Geometry check sheet. Reference: the model listing, model coordinates, mm. Give positions to 0.01 mm unless a question says otherwise; leave off trailing zeros. Write each loop counter-clockwise with the first axis right and the second up, starting at its lowest first coordinate (ties: lowest second). Pieces come first, ordered by that corner, then holes. Notation, with made-up numbers: (82.25, 17.5) -> (126.25, 17.5) arc R8 ccw to (126.25, 30.5) -> close; hole circle Ø11 at (30, -21). An arc over 180 degrees is marked (long way). One line per item, written item: value.
from build123d import *


with BuildPart() as part:
    # Esquisse1 → Révolution1 (revolve)
    with BuildSketch(Plane(origin=(0, 0, 0), x_dir=(-1, 0, 0), z_dir=(0, 0, -1)), mode=Mode.PRIVATE) as r_volution1_sk:
        with BuildLine():
            Line((-2.5, -1.85), (-2.5, 1.85))
            ThreePointArc((-2.5, 1.85), (-2.543933983, 1.956066017), (-2.65, 2))
            Line((-2.65, 2), (-2.95, 2))
            Line((-2.95, 2), (-2.95, 1.85))
            Line((-2.95, 1.85), (-4.55, 1.85))
            Line((-4.55, 1.85), (-4.55, 2))
            Line((-4.55, 2), (-4.85, 2))
            ThreePointArc((-4.85, 2), (-4.956066017, 1.956066017), (-5, 1.85))
            Line((-5, 1.85), (-5, -1.85))
            ThreePointArc((-5, -1.85), (-4.956066017, -1.956066017), (-4.85, -2))
            Line((-4.85, -2), (-4.55, -2))
            Line((-4.55, -2), (-4.55, -1.85))
            Line((-4.55, -1.85), (-2.95, -1.85))
            Line((-2.95, -1.85), (-2.95, -2))
            Line((-2.95, -2), (-2.65, -2))
            ThreePointArc((-2.65, -2), (-2.543933983, -1.956066017), (-2.5, -1.85))
        make_face()
    revolve(r_volution1_sk.sketch.rotate(Axis((0, -2.003446066, 0), (0, 1, 0)), 270), axis=Axis((0, -2.003446066, 0), (0, 1, 0)))


solid = part.part
1) Depth check by flat-ended pin: pin 1 Ø3 at (x, z) = (0, 0) entering from +Y. Enter the tip coordinate at first touch or a pass-through.
Verdict:
pin 1: through
2) Mould release check, pull along X, two halves, no side actions. Record for faces 1 (the flat face through (-3, -1.85, 1)), 2 (the cylindrical face through (-2.44, 0.03, -0.54)), 3 (the cylindrical face through (-4.88, -0.03, -1.08)): released by +X, released by -X, zero draft, split by the parting line, or undercut.
Verdict:
face 1: undercut
face 2: undercut
face 3: split by the parting line
3) Scan lines: probe 1 along X at (y, z) = (1.95, 0); probe 2 along Z at (x, y) = (-0.25, -0.5); probe 3 along Z at (x, y) = (-0.75, 0.5). Record each from-to range of solid material in increasing order.
Verdict:
probe 1: -4.96 to -4.55, -2.95 to -2.54, 2.54 to 2.95, 4.55 to 4.96
probe 2: -4.99 to -2.49, 2.49 to 4.99
probe 3: -4.94 to -2.38, 2.38 to 4.94
4) Sectioned sample at C-C on y = 0.55. Record the cut outline in (x, z), plus the area to 3 significant figures.
Verdict:
outline: circle Ø10 at (0, 0); hole circle Ø5 at (0, 0)
area: 58.9 mm^2
